```python
from build123d import *

# Parameters (mm, degrees)
F0_R            = 45
F0_R_2          = 33
F1_DEPTH        = 17
F2_R            = 5
F3_DEPTH        = 0.5
F3_COPIES_COUNT = 6
F6_DEPTH        = 10
F8_COUNT        = 6


# Not quite as in the source:
# - a pattern or mirror of a feature is missing from the dataset's text; its kind, count and spacing are read off the source's solid


with BuildPart() as f1:
    # F0 (on Front) → F1 (new body)
    with BuildSketch(Plane.XZ):
        Circle(F0_R)
        Circle(F0_R_2, mode=Mode.SUBTRACT)
    extrude(amount=F1_DEPTH)

    # F2 (on Front) → F3 (cut)
    with BuildSketch(Plane.XZ):
        with Locations((0, 39)):
            Circle(F2_R)
    f3 = extrude(amount=F3_DEPTH, mode=Mode.SUBTRACT)

    # F3_copies: F3 ×6 about axis
    f3_copies_axis = Axis((0, 0, 0), (0, 1, 0))
    for i in range(1, F3_COPIES_COUNT):
        add(f3.rotate(f3_copies_axis, i * 360 / F3_COPIES_COUNT), mode=Mode.SUBTRACT)

    # F5 (on face) → F6 (cut)
    with BuildSketch(Plane.XZ.offset(17)):
        with BuildLine():
            Line((-30.5409561082, 12.5), (-43.2290411645, 12.5))
            ThreePointArc((-43.2290411645, 12.5), (-45, 0), (-43.2290411645, -12.5))
            Line((-43.2290411645, -12.5), (-30.5409561082, -12.5))
            ThreePointArc((-30.5409561082, -12.5), (-33, 0), (-30.5409561082, 12.5))
        make_face()
    f6 = extrude(amount=-F6_DEPTH, mode=Mode.SUBTRACT)

    # F8: F6 ×6 about axis
    f8_axis = Axis((0, -20.116, 0), (0, -1, 0))
    for i in range(1, F8_COUNT):
        add(f6.rotate(f8_axis, i * 360 / F8_COUNT), mode=Mode.SUBTRACT)


solid = f1.part
```
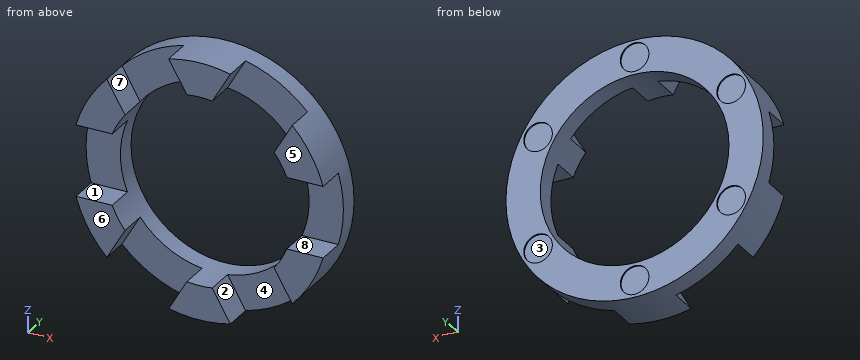
The model under review builds one solid part; all positions refer to its coordinate system, in mm. Face numbers are marked on the shaded views. A direction names the side the tool comes from. Round coordinates to 2 decimals unless told otherwise and drop trailing zeros. Loops run counter-clockwise (first coordinate to the right, second up) from the corner with the lowest first, then second, coordinate; pieces in that order, holes last. Notation, with made-up numbers: (-6, 6) -> (28, 6) arc R26 ccw to (28, 22) -> close; hole circle Ø5 at (27.25, -19). An arc over 180 degrees is marked (long way). Answer in a Markdown table with one row per item.
1) Wall thickness on line 1 along Z through (x, y) = (0, -3.5); line 2 along Z through (x, y) = (-30, -7.75); line 3 along X through (y, z) = (-16, 14): over which ranges is each line inside the solid? List them lowest first.
Taken from the geometry:
| item | result |
|---|---|
| line 1 | z = -45 to -33, 33 to 45 |
| line 2 | z = -26.96 to -13.75, 13.75 to 26.96 |
| line 3 | x = -42.77 to -29.88, 29.88 to 42.77 |
2) Consider section A-A, the plane y = -15.25. Write out the cut boundary in (x, z).
Taken from the geometry:
| item | result |
|---|---|
| outline | (-43.23, -12.5) arc R45 ccw to (-32.44, -31.19) -> (-26.1, -20.2) arc R33 cw to (-30.54, -12.5) -> close; (-43.23, 12.5) -> (-30.54, 12.5) arc R33 cw to (-26.1, 20.2) -> (-32.44, 31.19) arc R45 ccw to start; (-10.79, -43.69) arc R45 ccw to (10.79, -43.69) -> (4.45, -32.7) arc R33 cw to (-4.45, -32.7) -> close; (-10.79, 43.69) -> (-4.45, 32.7) arc R33 cw to (4.45, 32.7) -> (10.79, 43.69) arc R45 ccw to start; (26.1, -20.2) -> (32.44, -31.19) arc R45 ccw to (43.23, -12.5) -> (30.54, -12.5) arc R33 cw to start; (26.1, 20.2) arc R33 cw to (30.54, 12.5) -> (43.23, 12.5) arc R45 ccw to (32.44, 31.19) -> close |
3) For pin 1 Ø8 at (x, z) = (-34, 20) entering from +Y; pin 2 Ø12 at (x, z) = (20.5, -31) entering from +Y; pin 3 Ø3 at (x, y) = (-2.5, -3) entering from -Z; pin 4 Ø8 at (x, y) = (-37, -14) entering from +Z, all flat-tipped, find the tip position at first contact; note any pin that passes through.
Taken from the geometry:
| item | result |
|---|---|
| pin 1 | stops at y = -0.5 |
| pin 2 | stops at y = 0 |
| pin 3 | stops at z = -44.99 |
| pin 4 | stops at z = 30.59 |
4) Tool access review of the marked faces 1, 2, 3, 4 and 5: name each direction out of +Z, -Z, +X, -X, +Y, -Y from which nothing blocks a thin tool from reaching the whole face with its end or side.
Taken from the geometry:
| item | result |
|---|---|
| face 1 | +X, -X, -Y |
| face 2 | +X, -Y |
| face 3 | +Y |
| face 4 | -Y |
| face 5 | +Z, -Z, +X, -X, -Y |
5) Consider section B-B, the plane x = 0. Write out the cut boundary in (y, z), plus the area to 3 significant figures.
Taken from the geometry:
| item | result |
|---|---|
| outline | (-17, -45) -> (0, -45) -> (0, -44) -> (-0.5, -44) -> (-0.5, -34) -> (0, -34) -> (0, -33) -> (-17, -33) -> close; (-17, 33) -> (0, 33) -> (0, 34) -> (-0.5, 34) -> (-0.5, 44) -> (0, 44) -> (0, 45) -> (-17, 45) -> close |
| area | 398 mm² |
6) Consider section D-D, the plane y = -2.5. Write out the cut boundary in (x, z), plus the area to 3 significant figures.
Taken from the geometry:
| item | result |
|---|---|
| outline | circle Ø90 at (0, 0); hole circle Ø66 at (0, 0) |
| area | 2,940 mm² |
7) Consider section C-C, the plane z = 0. Write out the cut boundary in (x, y).
Taken from the geometry:
| item | result |
|---|---|
| outline | (-45, -7) -> (-33, -7) -> (-33, 0) -> (-45, 0) -> close; (33, -7) -> (45, -7) -> (45, 0) -> (33, 0) -> close |
8) Draft analysis for pull direction Z (two halves, no side actions). For the marked faces 6, 7 and 8, state which applies: pulls with the +Z half, pulls with the -Z half, needs draft (parallel to the pull), parting line crosses it, or undercut.
Taken from the geometry:
| item | result |
|---|---|
| face 6 | needs draft |
| face 7 | pulls with the +Z half |
| face 8 | undercut |
